Source: CAD feature listing. Evaluate the final solid. Frame: model axes, mm. Face numbers are marked on the shaded views. A direction names the side the tool comes from. Round coordinates to 2 decimals unless told otherwise and drop trailing zeros. Order: outer loops, then holes, each group sorted by start corner. A loop starts at its lowest first (then second) coordinate and runs counter-clockwise, first axis right, second up. Notation, with made-up numbers: (74.25, -30) -> (124.25, -30) arc R20 ccw to (124.25, 9) -> close; hole circle Ø2 at (44, -34). An arc over 180 degrees is marked (long way). Answer as CSV lines item,"result".
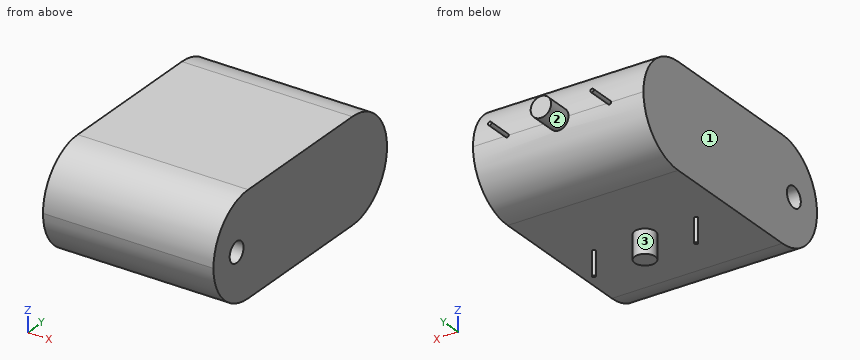
from build123d import *

# Parameters (mm, degrees)
EXTRUDE_1_DEPTH     = 30
SKETCH_2_R          = 3
CUT_EXTRUDE_1_DEPTH = 52
FILLET_1_R          = 15
FILLET_2_R          = 15
FILLET_3_R          = 15
FILLET_4_R          = 15
SKETCH_4_R          = 3
SKETCH_4_R_2        = 0.5
EXTRUDE_2_DEPTH     = 50
SKETCH_5_R          = 3
SKETCH_5_R_2        = 0.5
EXTRUDE_3_DEPTH     = 37


with BuildPart() as part:
    # 草图1 → 凸台-拉伸1 (new body)
    with BuildSketch(Plane.XY):
        Polygon((25, 0), (25, 42.5), (-25, 42.5), (-25, -32.5), (25, -32.5), align=None)
    extrude(amount=EXTRUDE_1_DEPTH)

    # 草图2 → 切除-拉伸1 (cut)
    with BuildSketch(Plane(origin=(25, 0, 0), x_dir=(0, 0, -1), z_dir=(1, 0, 0))):
        with Locations((-15, -22.5)):
            Circle(SKETCH_2_R)
    extrude(amount=-CUT_EXTRUDE_1_DEPTH, mode=Mode.SUBTRACT)

    # 圆角1
    fillet_1_edges = [part.edges().sort_by_distance(p)[0] for p in [
        (0, -32.5, 0),
    ]]
    fillet(fillet_1_edges, radius=FILLET_1_R)

    # 圆角2
    fillet_2_edges = [part.edges().sort_by_distance(p)[0] for p in [
        (0, -32.5, 30),
    ]]
    fillet(fillet_2_edges, radius=FILLET_2_R - 0.0001)  # a hair under: the kernel refuses the full size

    # 圆角3
    fillet_3_edges = [part.edges().sort_by_distance(p)[0] for p in [
        (0, 42.5, 30),
    ]]
    fillet(fillet_3_edges, radius=FILLET_3_R)

    # 圆角4
    fillet_4_edges = [part.edges().sort_by_distance(p)[0] for p in [
        (0, 42.5, 0),
    ]]
    fillet(fillet_4_edges, radius=FILLET_4_R - 0.0001)  # a hair under: the kernel refuses the full size

    # 草图4 → 凸台-拉伸2 (add)
    with BuildSketch(Plane(origin=(0, 0, 0), x_dir=(1, 0, 0), z_dir=(0, 1, 0))):
        with Locations((0, -15)):
            Circle(SKETCH_4_R)
        with Locations((15, -15)):
            Circle(SKETCH_4_R_2)
        with Locations((-15, -15)):
            Circle(SKETCH_4_R_2)
    extrude(amount=EXTRUDE_2_DEPTH)

    # 草图5 → 凸台-拉伸3 (add)
    with BuildSketch(Plane.XY.offset(30)):
        with Locations((0, 5)):
            Circle(SKETCH_5_R)
        with Locations((-15, 5)):
            Circle(SKETCH_5_R_2)
        with Locations((15, 5)):
            Circle(SKETCH_5_R_2)
    extrude(amount=-EXTRUDE_3_DEPTH)


solid = part.part
1. Section query B-B on z = 16.5. Return loops of the section in (x, y).
Results below:
outline,"(-25, -32.42) -> (25, -32.42) -> (25, -25.1) -> (-25, -25.1) -> close; (-25, -19.9) -> (25, -19.9) -> (25, 42.42) -> (2.6, 42.42) -> (2.6, 50) -> (-2.6, 50) -> (-2.6, 42.42) -> (-25, 42.42) -> close"
2. Line query: L1, parallel to Z at x = -19, y = -10.5; L2, parallel to Y at x = -21, z = 13; L3, parallel to Z at x = -6, y = -22. Output: solid intervals per line, ascending. Write a range as [from, to].
Results below:
L1,"[0, 30]"
L2,"[-32.37, -24.74], [-20.26, 42.37]"
L3,"[0.69, 12.04], [17.96, 29.31]"
3. Reachability of the marked faces 1, 2 and 3 from +Z, -Z, +X, -X, +Y, -Y: full face, straight path, thin tool, end or side. Return the list, or none.
Results below:
face 1,"+Z, -Z, -X, +Y, -Y"
face 2,"+Y"
face 3,"-Z"
4. Section query D-D on z = -1.5. Return loops of the section in (x, y), and give its area (3 significant figures).
Results below:
outline,"circle Ø1 at (-15, 5); circle Ø6 at (0, 5); circle Ø1 at (15, 5)"
area,"29.8 mm2"
5. Pin query (flat end, axial travel): pin 1 (1 mm diameter, centred on x = -17.5, z = 8, fed in from -Y). Return the tip coordinate at first contact, or that it passes through.
Results below:
pin 1,"y = -31.02"
6. Section query C-C on y = -22.5. Return loops of the section in (x, z), and give its area (3 significant figures).
Results below:
outline,"(-25, 0.86) -> (25, 0.86) -> (25, 12) -> (-25, 12) -> close; (-25, 18) -> (25, 18) -> (25, 29.14) -> (-25, 29.14) -> close"
area,"1,110 mm2"
